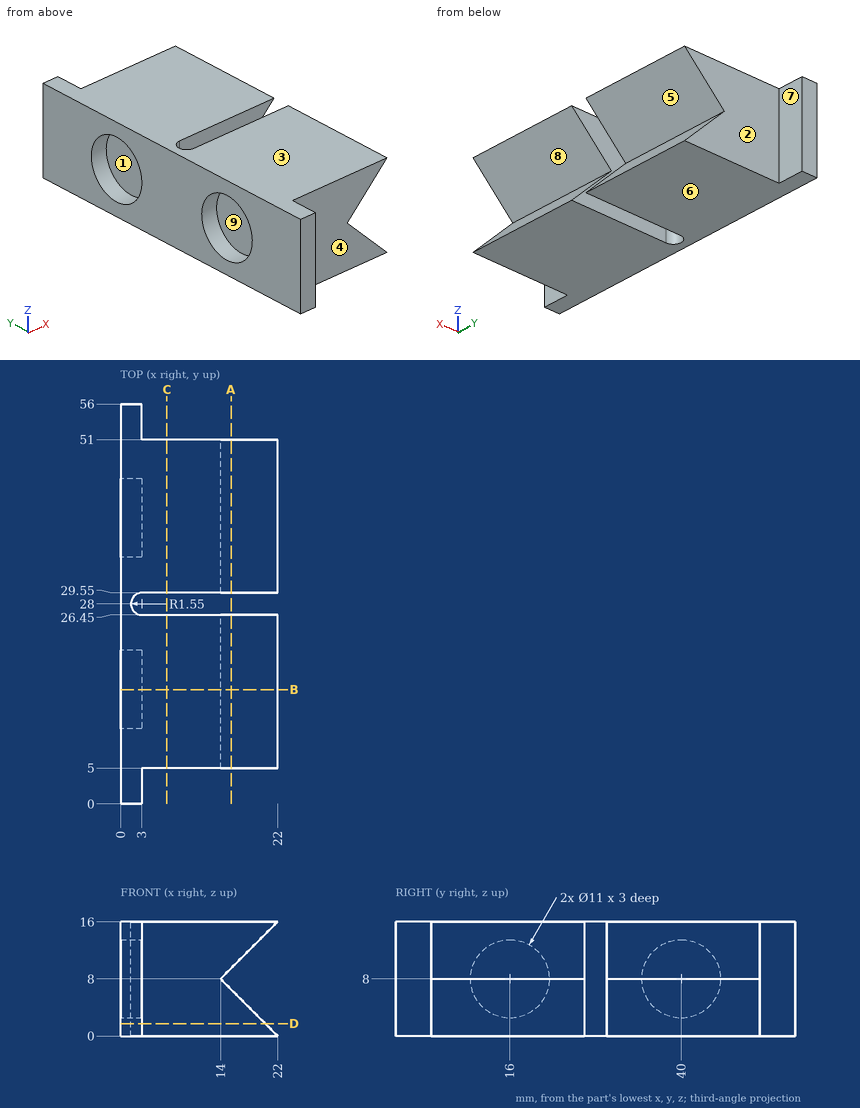
Answer from the drawing. Dimensions are ordinates in mm from the lowest x, y and z of the part. A direction names the side the tool comes from. Give positions to 0.01 mm unless a question says otherwise; leave off trailing zeros. Order: outer loops, then holes, each group sorted by start corner. A loop starts at its lowest first (then second) coordinate and runs counter-clockwise, first axis right, second up. Notation, with made-up numbers: (71.5, 56.25) - (115.5, 56.25) arc R18 ccw to (115.5, 61.25) - close; hole circle Ø9 at (11, 25). An arc over 180 degrees is marked (long way). One line per item, written item: value. Start each with the question number.
1. For a pull along Z with two mould halves and no side action, classify the marked faces 6, 7, 8 and 9 as released by +Z, released by -Z, zero draft, split by the parting line, or undercut.
2. Consider line 1 (Y direction, x = 0.95, z = 8); line 2 (Y direction, x = 2.3, z = 8); line 3 (Y direction, x = 4, z = 15.25). Determine where each line is inside the solid, lowest interval first.
3. Each of these flat-tipped pins is pushed along its axis until it touches: pin 1 Ø3.5 at (y, z) = (41, 6.5) entering from -X; pin 2 Ø8 at (x, z) = (10.5, 7.5) entering from -Y; pin 3 Ø1 at (y, z) = (49.5, 11) entering from +X. Where does it stop, or does it pass through?
4. Section C-C, the plane x = 6.5 is taken. Write down the section's boundary in (y, z).
5. Section D-D, the plane z = 1.75 is taken. Write down the section's boundary in (x, y).
6. Which of the six approach directions +Z, -Z, +X, -X, +Y, -Y give full straight-line access (tool end or side, diameter ignored) to the marked faces 1, 2, 3, 4 and 5?
7. Section B-B, the plane y = 16 is taken. Write down the section's boundary in (x, z).
8. Section A-A, the plane x = 15.5 is taken. Write down the section's boundary in (y, z).
Filled sheet:
1. face 6: released by -Z
1. face 7: zero draft
1. face 8: undercut
1. face 9: undercut
2. line 1: 0 to 10.5, 21.5 to 34.5, 45.5 to 56
2. line 2: 0 to 10.5, 21.5 to 26.62, 29.38 to 34.5, 45.5 to 56
2. line 3: 5 to 26.45, 29.55 to 51
3. pin 1: x = 3
3. pin 2: y = 5
3. pin 3: x = 17.5
4. outline: (5, 0) - (26.45, 0) - (26.45, 16) - (5, 16) - close; (29.55, 0) - (51, 0) - (51, 16) - (29.55, 16) - close
5. outline: (0, 0) - (3, 0) - (3, 5) - (20.25, 5) - (20.25, 26.45) - (3, 26.45) arc R1.55 cw to (3, 29.55) - (20.25, 29.55) - (20.25, 51) - (3, 51) - (3, 56) - (0, 56) - close
6. face 1: -X
6. face 2: +Z, -Z, +X, +Y
6. face 3: +Z, +X, -X, +Y, -Y
6. face 4: +Z, -Z, +X, -Y
6. face 5: +X, +Y, -Y
7. outline: (0, 0) - (22, 0) - (14, 8) - (22, 16) - (0, 16) - (0, 13.5) - (3, 13.5) - (3, 2.5) - (0, 2.5) - close
8. outline: (5, 0) - (26.45, 0) - (26.45, 6.5) - (5, 6.5) - close; (5, 9.5) - (26.45, 9.5) - (26.45, 16) - (5, 16) - close; (29.55, 0) - (51, 0) - (51, 6.5) - (29.55, 6.5) - close; (29.55, 9.5) - (51, 9.5) - (51, 16) - (29.55, 16) - close
